Input: dimensioned drawing with shaded views. Units: mm. Origin: part minimum x, y, z. Round coordinates to 2 decimals unless told otherwise and drop trailing zeros. Write each loop counter-clockwise with the first axis right and the second up, starting at its lowest first coordinate (ties: lowest second). Pieces come first, ordered by that corner, then holes. Notation, with made-up numbers: M -11,78 L 22,78 A18 ccw 22,107 Z; hole C 78.5,45.25 d11. An arc over 180 degrees is marked long. Answer as CSV lines item,"result". Start each with the question number.
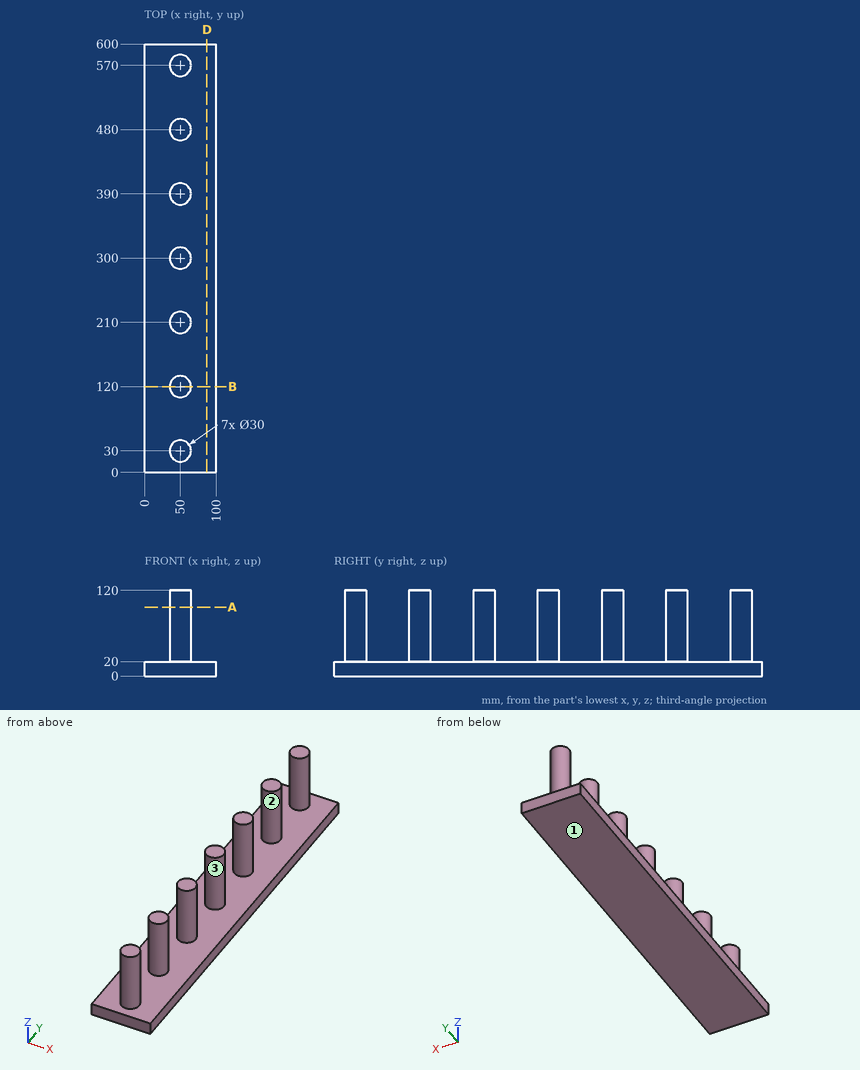
Item 1: Pin query (flat end, axial travel): pin 1 Ø1 at (x, y) = (64.5, 396) entering from +Z; pin 2 Ø6 at (y, z) = (219, 50) entering from +X; pin 3 Ø3 at (x, z) = (57.5, 64) entering from -Y. Return the tip coordinate at first contact, or that it passes through.
Item 2: Draft query along Y for the marked faces 1, 2 and 3. Return one class per face: +Y half, -Y half, draft (parallel to the pull), parting line (faces both ways), or undercut.
Item 3: Cut plane D-D, the plane x = 87. Return loops of the section in (y, z), plus the area to 3 significant figures.
Item 4: Line query: line 1 (Z direction, x = 44.5, y = 555.5); line 2 (X direction, y = 222, z = 56.5). Output: solid intervals per line, ascending. Write a range as [from, to].
Item 5: Cut plane A-A, the plane z = 96.5. Return loops of the section in (x, y).
Item 6: Cut plane B-B, the plane y = 120. Return loops of the section in (x, z), plus the area to 3 significant figures.
Results list:
1,pin 1,"z = 20"
1,pin 2,"x = 63.75"
1,pin 3,"y = 16.25"
2,face 1,"draft"
2,face 2,"undercut"
2,face 3,"undercut"
3,outline,"M 0,0 L 600,0 L 600,20 L 0,20 Z"
3,area,"12,000 mm²"
4,line 1,"[0, 20]"
4,line 2,"[41, 59]"
5,outline,"C 50,30 d30; C 50,120 d30; C 50,210 d30; C 50,300 d30; C 50,390 d30; C 50,480 d30; C 50,570 d30"
6,outline,"M 0,0 L 100,0 L 100,20 L 65,20 L 65,120 L 35,120 L 35,20 L 0,20 Z"
6,area,"5,000 mm²"
